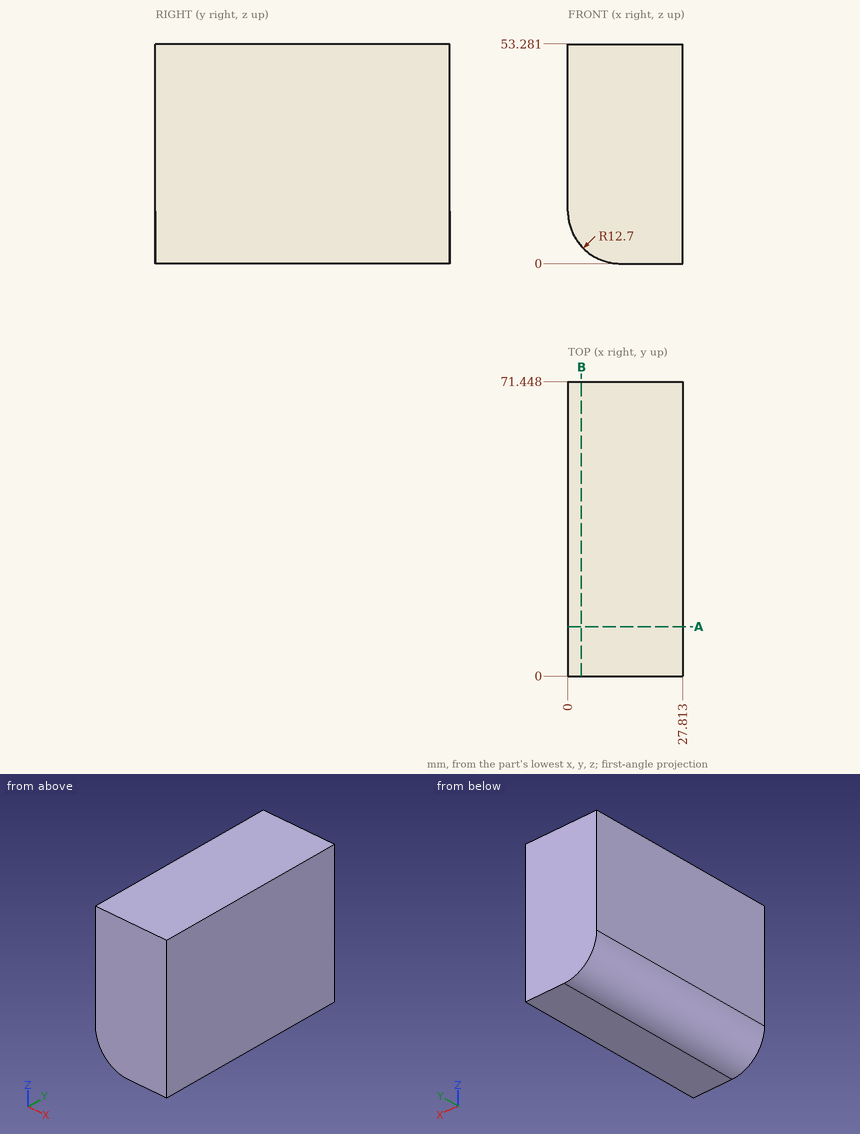
Input: dimensioned drawing with shaded views. Units: mm. Origin: part minimum x, y, z. Give positions to 0.01 mm unless a question says otherwise; leave off trailing zeros. Write each loop counter-clockwise with the first axis right and the second up, starting at its lowest first coordinate (ties: lowest second). Pieces come first, ordered by that corner, then holes. Notation, with made-up numbers: M 35.5,44 L 67.5,44 A27 cw 67.5,68 Z; hole C 24,64.25 d9. An arc over 180 degrees is marked long. Return JSON: item names as keys, results as strings. Group by question number.
1) Cut plane B-B, the plane x = 3.25. Output: boundary loops of the cut face in (y, z) (1 decimal).
2) Material intervals for line 1 along Z through (x, y) = (8.5, 14.5) (1 decimal); line 2 along Z through (x, y) = (3.75, 66); line 3 along X through (y, z) = (43, 9), sorted ascending. Write a range as [from, to].
3) Pin query (flat end, axial travel): P1, Ø3, axis at x = 3, y = 47, coming from the -Z side. Return the tip coordinate at first contact, or that it passes through.
4) Cut plane A-A, the plane y = 12. Output: boundary loops of the cut face in (x, z), plus the area to 3 significant figures.
Recorded:
{
 "1": {"outline": "M 0,4.2 L 71.4,4.2 L 71.4,53.3 L 0,53.3 Z"},
 "2": {"line 1": "z = [0.7, 53.3]", "line 2": "z = [3.69, 53.28]", "line 3": "x = [0.55, 27.81]"},
 "3": {"P1": "stops at z = 3"},
 "4": {"outline": "M 0,12.7 A12.7 ccw 12.7,0 L 27.81,0 L 27.81,53.28 L 0,53.28 Z", "area": "1,450 mm²"}
}
